Can you work these out from the drawing? Everything is in mm from the part's minimum corner. Give positions to 0.01 mm unless a question says otherwise; leave off trailing zeros. Write each loop counter-clockwise with the first axis right and the second up, starting at its lowest first coordinate (ties: lowest second). Pieces come first, ordered by that corner, then holes. Notation, with made-up numbers: (81, 70) -> (122, 70) arc R12 ccw to (122, 86) -> close; hole circle Ø11 at (77.25, 51). An arc over 180 degrees is marked (long way). Return JSON: item names as keys, results as strings.
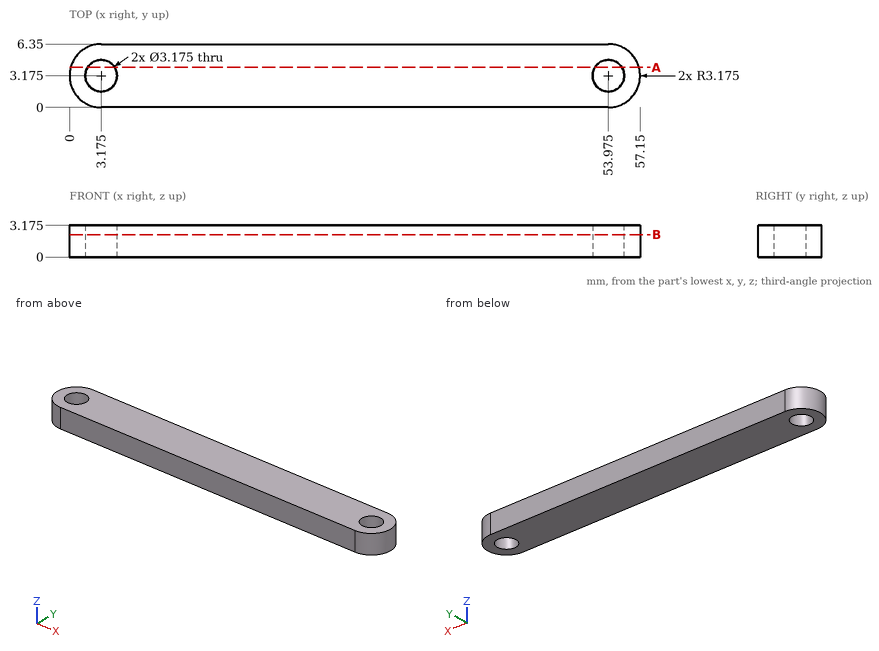
1. Suppose I cut it at B-B, the plane z = 2.25. Count the separate pieces of the cut face and the enclosed holes in it, and give its area (3 significant figures).
Taken from the geometry:
{"separate pieces": "1", "enclosed holes": "2", "area": "338 mm²"}
2. If I drill on line 1 (X direction, y = 3.25, z = 0.2); line 2 (X direction, y = 4.5, z = 1.8); line 3 (Y direction, x = 54, z = 1), over which ranges is the centre line in solid material (lowest first)? Write a range as [from, to].
Taken from the geometry:
{"line 1": "x = [0, 1.59], [4.76, 52.39], [55.56, 57.15]", "line 2": "x = [0.29, 2.3], [4.05, 53.1], [54.85, 56.86]", "line 3": "y = [0, 1.59], [4.76, 6.35]"}
3. Suppose I cut it at A-A, the plane y = 4. List the corners of the cut face in (x, z) for me (3 decimals).
Taken from the geometry:
{"outline": "(0.109, 0) -> (1.819, 0) -> (1.819, 3.175) -> (0.109, 3.175) -> close; (4.531, 0) -> (52.619, 0) -> (52.619, 3.175) -> (4.531, 3.175) -> close; (55.331, 0) -> (57.041, 0) -> (57.041, 3.175) -> (55.331, 3.175) -> close"}
4. For pin 1 Ø1 at (y, z) = (5.5, 0.5) entering from +X; pin 2 Ø3 at (x, y) = (13, 3.5) entering from -Z; pin 3 Ø1.9 at (x, y) = (3.175, 3.175) entering from -Z, each with a flat end and sliding along its axis, tell me the tip position at first contact or that it passes through.
Taken from the geometry:
{"pin 1": "stops at x = 56.57", "pin 2": "stops at z = 0", "pin 3": "passes through"}
